Autodesk Inventor part; units mm, degrees
ref_plane "YZ Plane" through (0, 0, 0) normal (1, 0, 0) x (0, 1, 0)
ref_plane "XZ Plane" through (0, 0, 0) normal (0, 1, 0) x (-1, 0, 0)
ref_plane "XY Plane" through (0, 0, 0) normal (0, 0, 1) x (1, 0, 0)
sketch "スケッチ1" plane through (0, 0, 0) normal (0, 0, 1) x (1, 0, 0)
  circle A0 centre (0, 0) radius 27.25
  line L0 (17.5, 17.5) -> (-17.5, 17.5)
  line L1 (-17.5, 17.5) -> (-17.5, -17.5)
  line L2 (-17.5, -17.5) -> (17.5, -17.5)
  line L3 (17.5, -17.5) -> (17.5, 17.5)
  line L4 (17.5, 17.5) -> (-17.5, -17.5) construction
  line L5 (-17.5, 17.5) -> (17.5, -17.5) construction
  line L6 (1, 17.5) -> (-1, 17.5)
  line L7 (-1, 17.5) -> (-1, -17.5)
  line L8 (-1, -17.5) -> (1, -17.5)
  line L9 (1, -17.5) -> (1, 17.5)
  line L10 (1, 17.5) -> (-1, -17.5) construction
  line L11 (-1, 17.5) -> (1, -17.5) construction
  point P0 (1, -17.5)
  point P1 (1, 17.5)
  point P2 (-1, 17.5)
  point P3 (-1, -17.5)
  dimension "d0" = 54.5
  dimension "d6" = 35
  dimension "d107" = 2
  dimension "d108" = 35
extrude "押し出し1" add sketch "スケッチ1" against normal blind 2 contours A0 | L9 L2 L7 L0
sketch "スケッチ2" plane through (0, 0, 0) normal (0, 0, 1) x (1, 0, 0)
  line L0 (0, 42.4511) -> (0, -37.5489)
  line L1 (38.0038, 0) -> (-41.9962, 0)
  line L2 (27.25, 42.0143) -> (27.25, -37.9857)
  circle A0 centre (0, 0) radius 27.25
  line L3 (17.5, 17.5) -> (17.5, -17.5)
  line L4 (19.25, 25) -> (27.25, 25)
  line L5 (27.25, 25) -> (27.25, -25)
  line L6 (27.25, -25) -> (19.25, -25)
  line L7 (19.25, -25) -> (19.25, 25)
  line L8 (19.25, 25) -> (27.25, -25) construction
  line L9 (27.25, 25) -> (19.25, -25) construction
  point P0 (17.5, 0)
  point P1 (23.25, 0)
  point P2 (19.25, 0)
  point P3 (27.25, 0)
  dimension "d13" = 9.75
  dimension "d14" = 8
  dimension "d15" = 50
  dimension "d19" = 54.5
  dimension "d110" = 1.75
extrude "押し出し2" cut sketch "スケッチ2" against normal blind 10 contours L7 L4 L2 A0 | A0 L1 L7 picked at (20.3822, 11.481)
mirror "ミラー1" about plane through (0, 0, 0) normal (1, 0, 0) of "押し出し2"
sketch "スケッチ8" plane through (0, 0, 0) normal (0, 0, 1) x (1, 0, 0)
  circle A0 centre (0, 0) radius 22.375
  circle A1 centre (0, 0) radius 27.25
  line L0 (0, 31.1603) -> (0, -30.8706)
  point P0 (0, 0)
  point P1 (0, 22.375)
  point P2 (0, -22.375)
  dimension "d112" = 44.75
  dimension "d113" = 54.5
hole "穴5" at (0, 22.375, 0) at (0, -22.375, 0) direction (0, 0, -1) diameter 6.6 end through all
properties part number "Part3_A_Y" material "鋼、軟鋼"
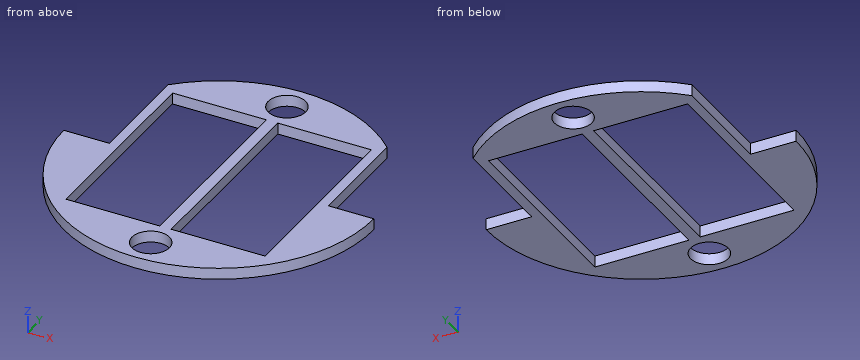
The model under review builds one solid part; all positions refer to its coordinate system, in mm. Round coordinates to 2 decimals unless told otherwise and drop trailing zeros. Loops run counter-clockwise (first coordinate to the right, second up) from the corner with the lowest first, then second, coordinate; pieces in that order, holes last. Notation, with made-up numbers: (36, -4) -> (84, -4) arc R21 ccw to (84, 13) -> close; hole circle Ø11 at (38.5, 4.5). An arc over 180 degrees is marked (long way). Answer as CSV lines item,"result".
1) Add section A-A on z = -1.65. Write out the cut boundary in (x, y) (3 decimals), plus the area to 3 significant figures.
Geometry results:
outline,"(-27.25, 0) arc R27.25 ccw to (27.25, 0) -> (19.25, 0) -> (19.25, 19.287) arc R27.25 ccw to (-19.25, 19.287) -> (-19.25, 0) -> close; hole (-17.5, -17.5) -> (-1, -17.5) -> (-1, 17.5) -> (-17.5, 17.5) -> close; hole circle Ø6.6 at (0, -22.375); hole circle Ø6.6 at (0, 22.375); hole (1, -17.5) -> (17.5, -17.5) -> (17.5, 17.5) -> (1, 17.5) -> close"
area,"897 mm²"
2) To check wall thickness, follow line 1 along Y through (x, z) = (0, -0.75) (3 decimals); line 2 along X through (y, z) = (-8.5, -0.8); line 3 along X through (y, z) = (-14, -1.55). State the ranges of each line that lie inside material, in increasing order. Write a range as from..to.
Geometry results:
line 1,"y = -27.25..-25.675, -19.075..19.075, 25.675..27.25"
line 2,"x = -25.89..-17.5, -1..1, 17.5..25.89"
line 3,"x = -23.38..-17.5, -1..1, 17.5..23.38"
3) For P1, Ø1, axis at x = 12, z = -1.5, coming from the -Y side; P2, Ø0.6, axis at x = 5.5, z = -1, coming from the +Y side; P3, Ø1, axis at x = -9.5, z = -1.5, coming from the -Y side, all flat-tipped, find the tip position at first contact; note any pin that passes through.
Geometry results:
P1,"stops at y = -24.7"
P2,"stops at y = 26.75"
P3,"stops at y = -25.72"
4) Add section B-B on y = 7.5. Write out the cut boundary in (x, z).
Geometry results:
outline,"(-19.25, -2) -> (-17.5, -2) -> (-17.5, 0) -> (-19.25, 0) -> close; (-1, -2) -> (1, -2) -> (1, 0) -> (-1, 0) -> close; (17.5, -2) -> (19.25, -2) -> (19.25, 0) -> (17.5, 0) -> close"
5) Add section D-D on y = -22.5. Write out the cut boundary in (x, z).
Geometry results:
outline,"(-15.37, -2) -> (-3.3, -2) -> (-3.3, 0) -> (-15.37, 0) -> close; (3.3, -2) -> (15.37, -2) -> (15.37, 0) -> (3.3, 0) -> close"
6) Add section C-C on x = 0. Write out the cut boundary in (y, z) (3 decimals), plus the area to 3 significant figures.
Geometry results:
outline,"(-27.25, -2) -> (-25.675, -2) -> (-25.675, 0) -> (-27.25, 0) -> close; (-19.075, -2) -> (19.075, -2) -> (19.075, 0) -> (-19.075, 0) -> close; (25.675, -2) -> (27.25, -2) -> (27.25, 0) -> (25.675, 0) -> close"
area,"82.6 mm²"
